```python
from build123d import *

# Parameters (mm, degrees)
F0_R     = 11
F0_W     = 60
F0_H     = 10
F1_DEPTH = 25
F2_DEPTH = 25
F3_START = 8
F0_R_2   = 9
F3_DEPTH = 17
F4_R     = 4
F5_DEPTH = 25


with BuildPart() as f1:
    # F0 (on Front) → F1 (new body)
    with BuildSketch(Plane.XZ):
        with BuildLine():
            ThreePointArc((16, 0), (0, 16), (-16, 0))
            Line((-16, 0), (-30, -60))
            Line((-30, -60), (30, -60))
            Line((30, -60), (16, 0))
        make_face()
        Circle(F0_R, mode=Mode.SUBTRACT)
        with Locations((0, -65)):
            Rectangle(F0_W, F0_H)
    extrude(amount=F1_DEPTH)

    # F0 (on Front) → F2 (join)
    with BuildSketch(Plane.XZ):
        with Locations((0, -65)):
            Rectangle(F0_W, F0_H)
    extrude(amount=-F2_DEPTH)

    # F0 (on Front) → F3 (join)
    with BuildSketch(Plane.XZ.offset(F3_START)):
        Circle(F0_R)
        Circle(F0_R_2, mode=Mode.SUBTRACT)
    extrude(amount=F3_DEPTH)

    # F4 (on face) → F5 (cut)
    with BuildSketch(Plane.XY.offset(-60)):
        with Locations((-14, 14)):
            Circle(F4_R)
        with Locations((14, 14)):
            Circle(F4_R)
    extrude(amount=-F5_DEPTH, mode=Mode.SUBTRACT)


solid = f1.part
```
Build history of the part. All positions in model axes, mm. A direction names the side the tool comes from. Give positions to 0.01 mm unless a question says otherwise; leave off trailing zeros. Loops run counter-clockwise (first coordinate to the right, second up) from the corner with the lowest first, then second, coordinate; pieces in that order, holes last.
Item 1: Flat gauge pins, fed straight in: pin 1 (3 mm diameter, centred on x = -20.5, y = 15.5, fed in from +Z); pin 2 (10.5 mm diameter, centred on x = -14, y = 14, fed in from -Z); pin 3 (10 mm diameter, centred on y = 2.5, z = -17, fed in from -X); pin 4 (1 mm diameter, centred on y = -5, z = -13.5, fed in from +X). Where does each tip first touch, or does it go through?
Answers follow:
pin 1: stops at z = -60
pin 2: stops at z = -70
pin 3: stops at x = -20.98
pin 4: stops at x = 19.27
Item 2: Which spindle directions (+Z, -Z, +X, -X, +Y, -Y) get a long thin tool onto all of the face, cutting with end or side? Do faces 1 (the face through (2, -8, -9)), 2 (the face through (-18, 14, -65)), 3 (the face through (0, 12, -60)). Say none if no direction does.
Answers follow:
face 1: +Y
face 2: +Z, -Z
face 3: +Z, +X, -X, +Y
Item 3: Slice it at A-A, the plane x = 0. List the corners of the cut face in (y, z).
Answers follow:
outline: (-25, -70) - (25, -70) - (25, -60) - (0, -60) - (0, -11) - (-8, -11) - (-8, -9) - (-25, -9) - close; (-25, 9) - (-8, 9) - (-8, 11) - (0, 11) - (0, 16) - (-25, 16) - close
Item 4: Drill centre lines: line 1 (Z direction, x = 0, y = -6); line 2 (Z direction, x = 0, y = -19); line 3 (Y direction, x = 14, z = -62). Where is each one in solid material? Low to high.
Answers follow:
line 1: z = -70 to -11, 11 to 16
line 2: z = -70 to -9, 9 to 16
line 3: y = -25 to 10, 18 to 25
Item 5: Slice it at D-D, the plane x = -14. List the corners of the cut face in (y, z), and give its area (3 significant figures).
Answers follow:
outline: (-25, -70) - (10, -70) - (10, -60) - (0, -60) - (0, 7.75) - (-25, 7.75) - close; (18, -70) - (25, -70) - (25, -60) - (18, -60) - close
area: 2,110 mm2
Item 6: Slice it at B-B, the plane y = -18. List the corners of the cut face in (x, z).
Answers follow:
outline: (-30, -70) - (30, -70) - (30, -60) - (16, 0) arc R16 ccw to (-16, 0) - (-30, -60) - close; hole circle Ø18 at (0, 0)
Item 7: Slice it at C-C, the plane z = 4.5. List the corners of the cut face in (x, y), and give its area (3 significant figures).
Answers follow:
outline: (-15.35, -25) - (-7.79, -25) - (-7.79, -8) - (-10.04, -8) - (-10.04, 0) - (-15.35, 0) - close; (7.79, -25) - (15.35, -25) - (15.35, 0) - (10.04, 0) - (10.04, -8) - (7.79, -8) - close
area: 342 mm2
Item 8: Pull direction X, two halves, no side cores. Call faces 4 (the face through (0, 0, -70)), 5 (the face through (-2.38, -3.94, -10.74)), 6 (the face through (0, -12, 16)): released by +X, released by -X, zero draft, split by the parting line, or undercut.
Answers follow:
face 4: zero draft
face 5: undercut
face 6: split by the parting line
